Geometry check sheet. Reference: drawing and pictorial views, mm from the part's lowest x, y, z. A direction names the side the tool comes from. Round coordinates to 2 decimals unless told otherwise and drop trailing zeros. Write each loop counter-clockwise with the first axis right and the second up, starting at its lowest first coordinate (ties: lowest second). Pieces come first, ordered by that corner, then holes. Notation, with made-up numbers: M 18.25,70.5 L 35.25,70.5 A17 cw 35.25,81.5 Z; hole C -14.75,68 d5. An arc over 180 degrees is marked long. Put each result on its own line as item: value. Start each with the question number.
(1) Mould release check, pull along Z, two halves, no side actions. Record for the marked faces 1, 2 and 3: pulls with the +Z half, pulls with the -Z half, needs draft (parallel to the pull), parting line crosses it, or undercut.
(2) Section check D-D on y = 19.5. Record the cut outline in (x, z), then the cut area to 3 significant figures.
(3) Gauge pin test, flat ends, axial feed: pin 1 (8 mm diameter, centred on x = 17.5, y = 22.5, fed in from -Z); pin 2 (2 mm diameter, centred on y = 21.5, z = 22.5, fed in from +X). Record the tip position at first contact, or that the pin passes through.
(4) Material ranges on probe 1 along Y at (x, z) = (1.2, 13); probe 2 along Y at (x, z) = (8.25, 27.95); probe 3 along Z at (x, y) = (14, 16.25), recorded low to high.
(5) Section check B-B on x = 8.25. Record the cut outline in (y, z).
(6) Section check A-A on y = 13. Record the cut outline in (x, z).
(7) Tool access check on the marked faces 4 and 5. Record the directions out of +Z, -Z, +X, -X, +Y, -Y that give a thin tool (end or side, any length) a straight path to the whole face; none if there is none.
(8) Section check C-C on z = 10.75. Record the cut outline in (x, y), then the cut area to 3 significant figures.
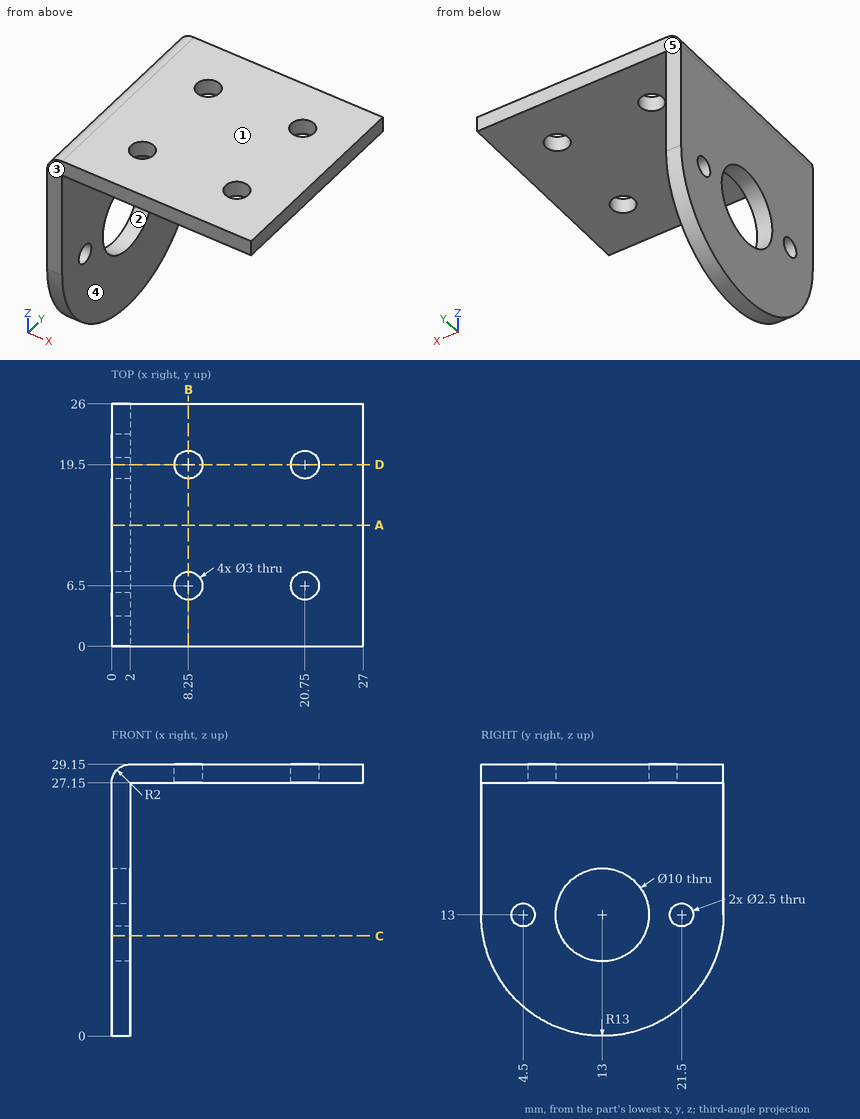
Answers follow:
1. face 1: pulls with the +Z half
1. face 2: undercut
1. face 3: needs draft
2. outline: M 0,1.74 L 2,1.74 L 2,27.15 L 6.75,27.15 L 6.75,29.15 L 2,29.15 A2 ccw 0,27.15 Z; M 9.75,27.15 L 19.25,27.15 L 19.25,29.15 L 9.75,29.15 Z; M 22.25,27.15 L 27,27.15 L 27,29.15 L 22.25,29.15 Z
2. area: 92.0 mm^2
3. pin 1: stops at z = 27.15
3. pin 2: stops at x = 2
4. probe 1: y = 0 to 3.25, 5.75 to 8, 18 to 20.25, 22.75 to 26
4. probe 2: y = 0 to 5, 8 to 18, 21 to 26
4. probe 3: z = 27.15 to 29.15
5. outline: M 0,27.15 L 5,27.15 L 5,29.15 L 0,29.15 Z; M 8,27.15 L 18,27.15 L 18,29.15 L 8,29.15 Z; M 21,27.15 L 26,27.15 L 26,29.15 L 21,29.15 Z
6. outline: M 0,0 L 2,0 L 2,8 L 0,8 Z; M 0,18 L 2,18 L 2,27.15 L 27,27.15 L 27,29.15 L 2,29.15 A2 ccw 0,27.15 Z
7. face 4: -Z, +X, +Y, -Y
7. face 5: +Z, -Z, +X, -X, +Y
8. outline: M 0,0.2 L 2,0.2 L 2,8.53 L 0,8.53 Z; M 0,17.47 L 2,17.47 L 2,25.8 L 0,25.8 Z
8. area: 33.4 mm^2
